from build123d import *

# Parameters (mm, degrees)
F0_W        = 60.96
F0_H        = 4.064
F1_DEPTH    = 60.96
F3_DEPTH    = 25.4
F4_R        = 2.0955
F5_DEPTH    = 6.35
F7_DEPTH    = 60.96
F8_T4_DEPTH = 53.34
F8_S5_R     = 30.988
F8_T6_DEPTH = 44
F8_S7_R     = 30.48
F8_T8_DEPTH = 44
F9_W        = 60.96
F9_H        = 4.064
F10_DEPTH   = 6.35
F11_W       = 3.175
F11_H       = 60.96
F12_DEPTH   = 7
F13_R       = 2.5
F14_DEPTH   = 3
F15_R       = 2.5
F16_DEPTH   = 3


# Not quite as in the source:
# - a fillet or chamfer that OpenCascade refuses, or shapes differently, is made with other operations: its cross-section is extruded or revolved along the edge and cut away or added


with BuildPart() as f1:
    # F0 (on Right) → F1 (new body)
    with BuildSketch(Plane.YZ):
        with Locations((2.5902520865, 22.5415869818)):
            Rectangle(F0_W, F0_H)
    extrude(amount=F1_DEPTH)

    # F2 (on face) → F3 (cut)
    with BuildSketch(Plane.XY.offset(24.5735869818)):
        with BuildLine():
            Line((16.002, -24.0797479135), (44.958, -24.0797479135))
            ThreePointArc((44.958, -24.0797479135), (51.934072902, -18.8638208155), (57.15, -11.8877479135))
            Line((57.15, -11.8877479135), (57.15, 17.0682520865))
            ThreePointArc((57.15, 17.0682520865), (51.934072902, 24.0443249885), (44.958, 29.2602520865))
            Line((44.958, 29.2602520865), (16.002, 29.2602520865))
            ThreePointArc((16.002, 29.2602520865), (9.0409528702, 24.0292992163), (3.81, 17.0682520865))
            Line((3.81, 17.0682520865), (3.81, -11.8877479135))
            ThreePointArc((3.81, -11.8877479135), (9.025927098, -18.8638208155), (16.002, -24.0797479135))
        make_face()
    extrude(amount=-F3_DEPTH, mode=Mode.SUBTRACT)

    # F4 (on face) → F5 (join)
    with BuildSketch(Plane.XY.offset(24.5735869818)):
        with Locations((55.88, -22.8097479135)):
            Circle(F4_R)
        with Locations((55.88, 27.9902520865)):
            Circle(F4_R)
        with Locations((5.08, -22.8097479135)):
            Circle(F4_R)
        with Locations((5.08, 27.9902520865)):
            Circle(F4_R)
    extrude(amount=F5_DEPTH)

    # F6 (on face) → F7 (join)
    with BuildSketch(Plane.XZ.offset(27.8897479135)):
        Polygon((30.48, -40.4504130182), (30.48, 20.5095869818), (0, 20.5095869818), align=None)
    extrude(amount=-F7_DEPTH)

    # F8: chamfer of 60.96 x 26.67 on 1 edges, made by hand


with BuildPart() as f8_tool2:
    # F8_s3 → F8_t4 (new body)
    with BuildSketch(Plane.XZ.offset(24.0797479135)):
        Polygon((3.81, 20.5095869818), (30.48, -40.4504130182), (30.48, 20.5095869818), align=None)
    extrude(amount=-F8_T4_DEPTH)

    # F8_s5 → F8_t6 (intersect, symmetric)
    with BuildSketch(Plane.XY.offset(-10)):
        with Locations((30.9527778056, 2.1174742809)):
            Circle(F8_S5_R)
    extrude(amount=F8_T6_DEPTH, both=True, mode=Mode.INTERSECT)

    # F8_s7 → F8_t8 (intersect, symmetric)
    with BuildSketch(Plane.XY.offset(-10)):
        with Locations((30.5785417886, 2.6887938751)):
            Circle(F8_S7_R)
    extrude(amount=F8_T8_DEPTH, both=True, mode=Mode.INTERSECT)


with BuildPart() as f1_1:
    add(f1.part)

    # F8_t1: cut F8_tool2
    add(f8_tool2.part, mode=Mode.SUBTRACT)

    # F9 (on face) → F10 (join)
    with BuildSketch(Plane.YZ.offset(60.96)):
        with Locations((2.5902520865, 22.5415869818)):
            Rectangle(F9_W, F9_H)
    extrude(amount=F10_DEPTH)

    # F11 (on face) → F12 (join)
    with BuildSketch(Plane(origin=(0, 0, 20.5095869818), x_dir=(1, 0, 0), z_dir=(0, 0, -1))):
        with Locations((65.7225, -2.5902520865)):
            Rectangle(F11_W, F11_H)
    extrude(amount=F12_DEPTH)

    # F13 (on face) → F14 (join)
    with BuildSketch(Plane(origin=(64.135, 0, 0), x_dir=(0, -1, 0), z_dir=(-1, 0, 0))):
        with Locations((-28.5702520865, 16.0095869818)):
            Circle(F13_R)
    extrude(amount=F14_DEPTH)

    # F15 (on face) → F16 (join)
    with BuildSketch(Plane(origin=(64.135, 0, 0), x_dir=(0, -1, 0), z_dir=(-1, 0, 0))):
        with Locations((23.3897479135, 16.0095869818)):
            Circle(F15_R)
    extrude(amount=F16_DEPTH)


solid = f1_1.part
Design review of the part built by this model. Coordinates are the model's own, in mm. A direction names the side the tool comes from. Round coordinates to 2 decimals unless told otherwise and drop trailing zeros. Loops run counter-clockwise (first coordinate to the right, second up) from the corner with the lowest first, then second, coordinate; pieces in that order, holes last. Notation, with made-up numbers: M -23,65 L 28,65 A23 cw 28,81 Z; hole C -3,20 d5. An arc over 180 degrees is marked long. Answer as a JSON object with one key per item and string values.
Item 1: The part is to be moulded in two halves that separate along X. For faces 1 (the cylindrical face through (6.047, -24.669, 27.704)), 2 (the flat face through (24, 33.07, 7)), say which applies: pulls with the +X half, pulls with the -X half, needs draft (parallel to the pull), parting line crosses it, or undercut.
Answer sheet:
{"face 1": "undercut", "face 2": "needs draft"}
Item 2: Machinability: for faces 3 (the cylindrical face through (62.66, -22.85, 13.57)), 4 (the flat face through (61.135, -23, 16)), 5 (the cylindrical face through (51.85, -18.95, 22.57)), 6 (the flat face through (27, -24.08, 0)), which of the approach directions +Z, -Z, +X, -X, +Y, -Y give a long, thin tool a straight path to every point of the face, cutting with its end or side? Answer none if there is none.
Answer sheet:
{"face 3": "none", "face 4": "-Z, +Y, -Y", "face 5": "+Z, -Z", "face 6": "+Z"}
Item 3: We need section D-D on x = 23. Give the boundary of the cut face in (y, z).
Answer sheet:
{"outline": "M -27.89,-25.49 L 33.07,-25.49 L 33.07,24.57 L 29.26,24.57 L 29.26,-23.35 L -24.08,-23.35 L -24.08,24.57 L -27.89,24.57 Z"}
Item 4: Clearance check with flat-ended pins moving along their axes: P1, Ø2, axis at x = 10.5, y = 7, coming from the -Z side; P2, Ø3.5, axis at y = 15, z = 15.5, coming from the -X side; P3, Ø1.9, axis at y = 31.5, z = -21, coming from the +X side. State where each tip first meets the part, or that it passes through.
Answer sheet:
{"P1": "stops at z = -2.49", "P2": "stops at x = 1.63", "P3": "stops at x = 30.48"}
Item 5: We need section B-B on x = 47. Give the boundary of the cut face in (y, z), and give its area (3 significant figures).
Answer sheet:
{"outline": "M -27.89,20.51 L -22.86,20.51 L -22.86,24.57 L -27.89,24.57 Z; M 28.04,20.51 L 33.07,20.51 L 33.07,24.57 L 28.04,24.57 Z", "area": "40.9 mm^2"}
Item 6: We need section A-A on y = 6.5. Give the boundary of the cut face in (x, z) (3 decimals).
Answer sheet:
{"outline": "M 0,20.51 L 30.48,-40.45 L 3.81,20.51 L 3.81,24.574 L 0,24.574 Z; M 57.15,20.51 L 64.135,20.51 L 64.135,13.51 L 67.31,13.51 L 67.31,24.574 L 57.15,24.574 Z"}
Item 7: Wall thickness on L1, parallel to X at y = 28, z = 25.5; L2, parallel to Z at x = 61, y = 8; L3, parallel to Y at x = 56, z = 25: over which ranges is each line inside the solid? List them lowest first. Write a range as from..to.
Answer sheet:
{"L1": "x = 2.98..7.18, 53.78..57.98", "L2": "z = 20.51..24.57", "L3": "y = -24.9..-20.72, 25.9..30.08"}
Item 8: We need section C-C on z = 6. Give the boundary of the cut face in (x, y), and give its area (3 significant figures).
Answer sheet:
{"outline": "M 7.25,-27.89 L 30.48,-27.89 L 30.48,-24.08 L 16,-24.08 A30.48 cw 10.16,-19.94 L 10.16,25.09 A30.99 cw 16,29.26 L 30.48,29.26 L 30.48,33.07 L 7.25,33.07 Z", "area": "354 mm^2"}
